Read the model definition and answer for the solid it produces. Units are mm, in the model's axes. A direction names the side the tool comes from. Round coordinates to 2 decimals unless told otherwise and drop trailing zeros. Loops run counter-clockwise (first coordinate to the right, second up) from the corner with the lowest first, then second, coordinate; pieces in that order, holes last. Notation, with made-up numbers: M 83.25,21 L 140.25,21 A8 ccw 140.25,28 Z; hole C 34.5,26 d4. An arc over 180 degrees is marked long. Write each question's results on one line, items separated by ' | '.
```python
from build123d import *

# Parameters (mm, degrees)
SKETCH1_R               = 1.65
SKETCH1_W               = 5.5
SKETCH1_H               = 10.5
BOSS_EXTRUDE1_DEPTH     = 1
SKETCH2_R               = 10
SKETCH2_R_2             = 1.65
SKETCH2_W               = 5.5
SKETCH2_H               = 10.5
BOSS_EXTRUDE2_DEPTH     = 4.2
SKETCH3_R               = 10
SKETCH3_R_2             = 1.65
BOSS_EXTRUDE3_DEPTH     = 3
SKETCH4_R               = 5
BOSS_EXTRUDE4_DEPTH     = 1
SKETCH5_R               = 3.9
BOSS_EXTRUDE5_DEPTH     = 7
SKETCH6_R               = 3
CUT_EXTRUDE1_DEPTH      = 10
CUT_EXTRUDE1_DEPTH_BACK = 4
CHAMFER1_SIZE           = 0.2


with BuildPart() as part:
    # Sketch1 → Boss-Extrude1 (new body)
    with BuildSketch(Plane(origin=(0, 0, 0), x_dir=(1, 0, 0), z_dir=(0, 1, 0))):
        with BuildLine():
            ThreePointArc((-11.832159566, 0), (0, -10), (11.832159566, 0))
            ThreePointArc((11.832159566, 0), (0, 10), (-11.832159566, 0))
        make_face()
        with Locations(Location((-6, 0, 0), (0, 0, 270))):
            Circle(SKETCH1_R, mode=Mode.SUBTRACT)
        with Locations(Location((6, 0, 0), (0, 0, 270))):
            Circle(SKETCH1_R, mode=Mode.SUBTRACT)
        Rectangle(SKETCH1_W, SKETCH1_H, mode=Mode.SUBTRACT)
    extrude(amount=BOSS_EXTRUDE1_DEPTH)

    # Sketch2 → Boss-Extrude2 (add)
    with BuildSketch(Plane(origin=(0, 1, 0), x_dir=(1, 0, 0), z_dir=(0, 1, 0))):
        with Locations(Location((0, 2, 0), (0, 0, 159.512684885))):
            Circle(SKETCH2_R)
        with Locations(Location((6, 0, 0), (0, 0, 270))):
            Circle(SKETCH2_R_2, mode=Mode.SUBTRACT)
        with Locations(Location((-6, 0, 0), (0, 0, 270))):
            Circle(SKETCH2_R_2, mode=Mode.SUBTRACT)
        Rectangle(SKETCH2_W, SKETCH2_H, mode=Mode.SUBTRACT)
    extrude(amount=BOSS_EXTRUDE2_DEPTH)

    # Sketch3 → Boss-Extrude3 (add)
    with BuildSketch(Plane(origin=(0, 5.2, 0), x_dir=(1, 0, 0), z_dir=(0, 1, 0))):
        with Locations(Location((0, 2, 0), (0, 0, 159.512684885))):
            Circle(SKETCH3_R)
        with Locations(Location((6, 0, 0), (0, 0, 270))):
            Circle(SKETCH3_R_2, mode=Mode.SUBTRACT)
        with Locations(Location((-6, 0, 0), (0, 0, 270))):
            Circle(SKETCH3_R_2, mode=Mode.SUBTRACT)
    extrude(amount=BOSS_EXTRUDE3_DEPTH)

    # Sketch4 → Boss-Extrude4 (add)
    with BuildSketch(Plane(origin=(0, 8.2, 0), x_dir=(1, 0, 0), z_dir=(0, 1, 0))):
        with Locations(Location((0, 0, 0), (0, 0, 13.762144757))):
            Circle(SKETCH4_R)
    extrude(amount=BOSS_EXTRUDE4_DEPTH)

    # Sketch5 → Boss-Extrude5 (add)
    with BuildSketch(Plane(origin=(0, 9.2, 0), x_dir=(1, 0, 0), z_dir=(0, 1, 0))):
        with Locations(Location((0, 0, 0), (0, 0, 270))):
            Circle(SKETCH5_R)
    extrude(amount=BOSS_EXTRUDE5_DEPTH)

    # Sketch6 → Cut-Extrude1 (cut, two sides)
    with BuildSketch(Plane(origin=(0, 9.2, 0), x_dir=(1, 0, 0), z_dir=(0, 1, 0))) as cut_extrude1_sk:
        with Locations(Location((-6, 0, 0), (0, 0, 56.251011404))):
            Circle(SKETCH6_R)
        with Locations(Location((6, 0, 0), (0, 0, 123.748988596))):
            Circle(SKETCH6_R)
    extrude(amount=CUT_EXTRUDE1_DEPTH, mode=Mode.SUBTRACT)
    extrude(cut_extrude1_sk.sketch, amount=-CUT_EXTRUDE1_DEPTH_BACK, mode=Mode.SUBTRACT)

    # Chamfer1
    chamfer1_edges = [part.edges().sort_by_distance(p)[0] for p in [
        (9.367496998, 8.2, 1.5),
    ]]
    chamfer(chamfer1_edges, length=CHAMFER1_SIZE)


solid = part.part
```
1. Given P1, Ø4, axis at y = 10, z = 4, coming from the -X side; P2, Ø5, axis at x = -7, z = 0, coming from the +Y side; P3, Ø1, axis at x = -8.5, y = 3.5, coming from the -Z side, each flat-ended and moving along its own axis, determine where each tip first touches the part or whether it passes through.
Completed:
P1: stops at x = -8.35 | P2: stops at y = 8.2 | P3: stops at z = -8
2. Find section B-B, the plane x = 0. Give the vertices of the cut face in (y, z).
Completed:
outline: M 0,-10 L 1,-10 L 1,-12 L 8,-12 L 8.2,-11.8 L 8.2,-5 L 9.2,-5 L 9.2,-3.9 L 16.2,-3.9 L 16.2,3.9 L 9.2,3.9 L 9.2,5 L 8.2,5 L 8.2,7.8 L 8,8 L 1,8 L 1,10 L 0,10 L 0,5.25 L 5.2,5.25 L 5.2,-5.25 L 0,-5.25 Z
3. Find section C-C, the plane z = -2. Give the vertices of the cut face in (x, y).
Completed:
outline: M -11.31,0 L -2.75,0 L -2.75,5.2 L 2.75,5.2 L 2.75,0 L 11.31,0 L 11.31,1 L 10,1 L 10,8 L 9.8,8.2 L 8.24,8.2 L 8.24,5.2 L 3.76,5.2 L 3.76,9.2 L 3.35,9.2 L 3.35,16.2 L -3.35,16.2 L -3.35,9.2 L -3.76,9.2 L -3.76,5.2 L -8.24,5.2 L -8.24,8.2 L -9.8,8.2 L -10,8 L -10,1 L -11.31,1 Z
4. Find the intervals of material crossed by L1, parallel to X at y = 1.5, z = 0; L2, parallel to Y at x = -9.75, z = 3.25; L3, parallel to Y at x = 9.25, z = -2.5, in increasing order.
Completed:
L1: x = -9.8 to -7.65, -4.35 to -2.75, 2.75 to 4.35, 7.65 to 9.8 | L2: y = 0 to 1 | L3: y = 0 to 8.2
5. Find section A-A, the plane y = 7.25. Give the vertices of the cut face in (x, z), then the cut area to 3 significant figures.
Completed:
outline: C 0,-2 d20; hole C -6,0 d6; hole C 6,0 d6 | area: 258 mm2
6. Find section D-D, the plane y = 14.5. Give the vertices of the cut face in (x, z), then the cut area to 3 significant figures.
Completed:
outline: M -3.52,-1.68 A3.9 ccw 3.52,-1.68 A3 cw 3.52,1.68 A3.9 ccw -3.52,1.68 A3 cw Z | area: 43.7 mm2
7. Determine the mould class of faces 1 (the face through (6, 5.2, -2)), 2 (the face through (-3, 0, 0)), 3 (the face through (-4, 5.2, 0)), 4 (the face through (-0.2, 0.5, 10)) for opening direction X: released by +X, released by -X, zero draft, split by the parting line, or undercut.
Completed:
face 1: undercut | face 2: zero draft | face 3: undercut | face 4: split by the parting line
8. Which of the six approach directions +Z, -Z, +X, -X, +Y, -Y give full straight-line access (tool end or side, diameter ignored) to faces 5 (the face through (0.1, 12.7, -3.9)), 6 (the face through (-0.1, 12.7, 3.9)), 7 (the face through (5.447, 4.451, -10.386)), 8 (the face through (0.2, 0.5, -10)), 9 (the face through (2.75, 3, 0))?
Completed:
face 5: -Z, +Y | face 6: +Z, +Y | face 7: +Y | face 8: -Z, -Y | face 9: -Y
